Could you check a few things on this model? Use its own coordinates, in mm. Face numbers are marked on the shaded views. A direction names the side the tool comes from. Round coordinates to 2 decimals unless told otherwise and drop trailing zeros. Write each loop counter-clockwise with the first axis right and the second up, starting at its lowest first coordinate (ties: lowest second). Pieces come first, ordered by that corner, then holes. Notation, with made-up numbers: (58.25, -8.75) -> (73.25, -8.75) arc R16 cw to (73.25, 11.25) -> close; hole circle Ø10 at (-24, -15). An arc over 180 degrees is marked (long way). Return JSON: item names as keys, results as strings.
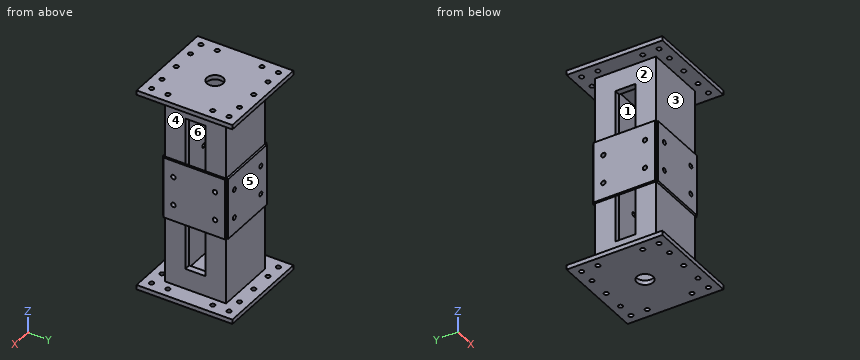
from build123d import *

# Parameters (mm, degrees)
SKETCH_1_W          = 300
SKETCH_1_H          = 300
EXTRUDE_1_DEPTH     = 956
SKETCH_2_W          = 240
SKETCH_2_H          = 240
CUT_EXTRUDE_1_DEPTH = 1046.913954396
SKETCH_4_W          = 756
SKETCH_4_H          = 100
CUT_EXTRUDE_2_DEPTH = 1046.913954396
SKETCH_5_W          = 470
SKETCH_5_H          = 470
EXTRUDE_2_DEPTH     = 22
SKETCH_6_W          = 470
SKETCH_6_H          = 470
EXTRUDE_3_DEPTH     = 22
SKETCH_7_R          = 11
CUT_EXTRUDE_3_DEPTH = 1139.617582861
SKETCH_9_W          = 300
SKETCH_9_H          = 300
EXTRUDE_4_DEPTH     = 10
SKETCH_10_W         = 300
SKETCH_10_H         = 300
EXTRUDE_5_DEPTH     = 10
SKETCH_11_W         = 300
SKETCH_11_H         = 300
EXTRUDE_6_DEPTH     = 10
SKETCH_12_W         = 300
SKETCH_12_H         = 300
EXTRUDE_7_DEPTH     = 10
SKETCH_13_R         = 11
CUT_EXTRUDE_4_DEPTH = 1123.824118017
SKETCH_14_R         = 11
CUT_EXTRUDE_5_DEPTH = 1123.824118017
SKETCH_15_R         = 40
CUT_EXTRUDE_6_DEPTH = 1139.617582861


with BuildPart() as part:
    # 草图1 → 拉伸1 (new body)
    with BuildSketch(Plane.XY):
        with Locations((150, 150)):
            Rectangle(SKETCH_1_W, SKETCH_1_H)
    extrude(amount=EXTRUDE_1_DEPTH)

    # 草图2 → 切除-拉伸1 (cut, through all)
    with BuildSketch(Plane.XY.offset(956)):
        with Locations((150, 150)):
            Rectangle(SKETCH_2_W, SKETCH_2_H)
    extrude(amount=-CUT_EXTRUDE_1_DEPTH, mode=Mode.SUBTRACT)

    # 草图4 → 切除-拉伸2 (cut, through all)
    with BuildSketch(Plane.ZY):
        with Locations((478, 150)):
            Rectangle(SKETCH_4_W, SKETCH_4_H)
    extrude(amount=-CUT_EXTRUDE_2_DEPTH, mode=Mode.SUBTRACT)

    # 草图5 → 拉伸2 (add)
    with BuildSketch(Plane.XY.offset(956)):
        with Locations((150, 150)):
            Rectangle(SKETCH_5_W, SKETCH_5_H)
    extrude(amount=EXTRUDE_2_DEPTH)

    # 草图6 → 拉伸3 (add)
    with BuildSketch(Plane(origin=(0, 0, 0), x_dir=(-1, 0, 0), z_dir=(0, 0, -1))):
        with Locations((-150, 150)):
            Rectangle(SKETCH_6_W, SKETCH_6_H)
    extrude(amount=EXTRUDE_3_DEPTH)

    # 草图7 → 切除-拉伸3 (cut, through all)
    with BuildSketch(Plane.XY.offset(978)):
        with Locations((-40, -40)):
            Circle(SKETCH_7_R)
        with Locations((40, -40)):
            Circle(SKETCH_7_R)
        with Locations((150, -40)):
            Circle(SKETCH_7_R)
        with Locations((260, -40)):
            Circle(SKETCH_7_R)
        with Locations((340, -40)):
            Circle(SKETCH_7_R)
        with Locations((-40, 340)):
            Circle(SKETCH_7_R)
        with Locations((40, 340)):
            Circle(SKETCH_7_R)
        with Locations((150, 340)):
            Circle(SKETCH_7_R)
        with Locations((260, 340)):
            Circle(SKETCH_7_R)
        with Locations((340, 340)):
            Circle(SKETCH_7_R)
        with Locations((-40, 40)):
            Circle(SKETCH_7_R)
        with Locations((-40, 260)):
            Circle(SKETCH_7_R)
        with Locations((340, 40)):
            Circle(SKETCH_7_R)
        with Locations((340, 260)):
            Circle(SKETCH_7_R)
    extrude(amount=-CUT_EXTRUDE_3_DEPTH, mode=Mode.SUBTRACT)

    # 草图9 → 拉伸4 (add)
    with BuildSketch(Plane(origin=(0, 300, 0), x_dir=(1, 0, 0), z_dir=(0, 1, 0))):
        with Locations((150, -478)):
            Rectangle(SKETCH_9_W, SKETCH_9_H)
    extrude(amount=EXTRUDE_4_DEPTH)

    # 草图10 → 拉伸5 (add)
    with BuildSketch(Plane.XZ):
        with Locations((150, 478)):
            Rectangle(SKETCH_10_W, SKETCH_10_H)
    extrude(amount=EXTRUDE_5_DEPTH)

    # 草图11 → 拉伸6 (add)
    with BuildSketch(Plane(origin=(300, 0, 0), x_dir=(0, 0, -1), z_dir=(1, 0, 0))):
        with Locations((-478, 150)):
            Rectangle(SKETCH_11_W, SKETCH_11_H)
    extrude(amount=EXTRUDE_6_DEPTH)

    # 草图12 → 拉伸7 (add)
    with BuildSketch(Plane.ZY):
        with Locations((478, 150)):
            Rectangle(SKETCH_12_W, SKETCH_12_H)
    extrude(amount=EXTRUDE_7_DEPTH)

    # 草图13 → 切除-拉伸4 (cut, through all)
    with BuildSketch(Plane.ZY.offset(10)):
        with Locations((408, 48)):
            Circle(SKETCH_13_R)
        with Locations((408, 252)):
            Circle(SKETCH_13_R)
        with Locations((548, 252)):
            Circle(SKETCH_13_R)
        with Locations((548, 48)):
            Circle(SKETCH_13_R)
    extrude(amount=-CUT_EXTRUDE_4_DEPTH, mode=Mode.SUBTRACT)

    # 草图14 → 切除-拉伸5 (cut, through all)
    with BuildSketch(Plane(origin=(0, 310, 0), x_dir=(1, 0, 0), z_dir=(0, 1, 0))):
        with Locations(Location((48, -548, 0), (0, 0, 270))):
            Circle(SKETCH_14_R)
        with Locations(Location((252, -548, 0), (0, 0, 270))):
            Circle(SKETCH_14_R)
        with Locations(Location((252, -408, 0), (0, 0, 270))):
            Circle(SKETCH_14_R)
        with Locations(Location((48, -408, 0), (0, 0, 270))):
            Circle(SKETCH_14_R)
    extrude(amount=-CUT_EXTRUDE_5_DEPTH, mode=Mode.SUBTRACT)

    # 草图15 → 切除-拉伸6 (cut, through all)
    with BuildSketch(Plane.XY.offset(978)):
        with Locations((150, 150)):
            Circle(SKETCH_15_R)
    extrude(amount=-CUT_EXTRUDE_6_DEPTH, mode=Mode.SUBTRACT)


solid = part.part
1) I want a section at A-A, the plane z = 162. Please give me the cut outline in (x, y), and give its area (3 significant figures).
Return value:
{"outline": "(0, 0) -> (300, 0) -> (300, 100) -> (270, 100) -> (270, 30) -> (30, 30) -> (30, 100) -> (0, 100) -> close; (0, 200) -> (30, 200) -> (30, 270) -> (270, 270) -> (270, 200) -> (300, 200) -> (300, 300) -> (0, 300) -> close", "area": "26,400 mm²"}
2) If I drill on probe 1 along X at (y, z) = (3, 548); probe 2 along Y at (x, z) = (150, 966.25); probe 3 along Y at (x, z) = (4.5, 408), over which ranges is the centre line in solid material (lowest first)? Write a range as [from, to].
Return value:
{"probe 1": "[-10, 37], [59, 241], [263, 310]", "probe 2": "[-85, -51], [-29, 110], [190, 329], [351, 385]", "probe 3": "[-10, 37], [59, 100], [200, 241], [263, 310]"}
3) I want a section at C-C, the plane y = 340. Count the separate pieces of the cut face and the enclosed holes in it, and give its area (3 significant figures).
Return value:
{"separate pieces": "12", "enclosed holes": "0", "area": "15,800 mm²"}
4) For the marked faces 4, 5 and 6, which set-ups out of +Z, -Z, +X, -X, +Y, -Y let a thin tool reach every point of the face, with its end or its side?
Return value:
{"face 4": "+X, +Y, -Y", "face 5": "+X, -X, +Y", "face 6": "none"}
5) Will these pins go through, and if not, where does the flat tip stop? pin 1 Ø8 at (y, z) = (-6.5, 532.5) entering from +X; pin 2 Ø17.5 at (y, z) = (48, 548) entering from -X; pin 3 Ø1 at (y, z) = (275, 310.5) entering from -X; pin 4 Ø3 at (x, z) = (266.5, 280) entering from +Y.
Return value:
{"pin 1": "x = 300", "pin 2": "through", "pin 3": "x = 0", "pin 4": "y = 300"}
6) Thinking about a two-plate mould opening in X: for the marked faces 1, 2 and 3, which applies, pulls with the +X half, pulls with the -X half, needs draft (parallel to the pull), parting line crosses it, or undercut?
Return value:
{"face 1": "undercut", "face 2": "pulls with the -X half", "face 3": "needs draft"}
7) I want a section at B-B, the plane x = 98.5. Please give me the cut outline in (y, z), and give its area (3 significant figures).
Return value:
{"outline": "(-85, -22) -> (385, -22) -> (385, 0) -> (300, 0) -> (300, 328) -> (310, 328) -> (310, 628) -> (300, 628) -> (300, 956) -> (385, 956) -> (385, 978) -> (-85, 978) -> (-85, 956) -> (0, 956) -> (0, 628) -> (-10, 628) -> (-10, 328) -> (0, 328) -> (0, 0) -> (-85, 0) -> close; hole (30, 0) -> (270, 0) -> (270, 956) -> (30, 956) -> close", "area": "84,000 mm²"}
